Autodesk Fusion 360 part; units mm, degrees
sketch "Sketch1" plane through (0, 0, 0) normal (0, 1, 0) x (1, 0, 0)
  line L0 (0, 0) -> (79, 0)
  line L1 (79, 0) -> (79, -80)
  line L2 (79, -80) -> (0, -80)
  line L3 (0, -80) -> (0, 0)
  dimension "d1" = 79
  dimension "d2" = 80
extrude "Extrude1" add sketch "Sketch1" along normal blind 5
sketch "Sketch2" plane through (0, 5, 0) normal (0, 1, 0) x (-1, 0, 0)
  line L0 (0, 80) -> (-79, 80)
  line L1 (-79, 80) -> (-79, 0)
  line L2 (-79, 0) -> (0, 0)
  line L3 (0, 0) -> (0, 80)
  point P0 (-14, 77.5)
  dimension "d5" = 14
  dimension "d6" = 2.5
hole "Hole1" at (14, 5, 77.5) direction (0, -1, 0) diameter 2 end through all counterbore diameter 4.4 counterbore depth 2.2
pattern_linear "R-Pattern1" count 1 spacing 0 along (0, 0, -1) count 4 spacing 17 along (1, 0, 0) of "Hole1"
Model file for the job. Use its own axes, mm. A direction names the side the tool comes from. Round coordinates to 2 decimals unless told otherwise and drop trailing zeros. Write each loop counter-clockwise with the first axis right and the second up, starting at its lowest first coordinate (ties: lowest second). Pieces come first, ordered by that corner, then holes. Notation, with made-up numbers: (39, 38.5) - (43, 38.5) arc R16 cw to (43, 61.5) - close; hole circle Ø5 at (61, 16). An arc over 180 degrees is marked (long way). One line per item, written item: value.
(1) Two-plate mould, pull along Z, no slides. Class faces 1 (the flat face through (79, 2, 39)), 2 (the cylindrical face through (47.324, 1.38, 76.763)), 3 (the flat face through (40, 2, 80)): pulls with the +Z half, pulls with the -Z half, needs draft (parallel to the pull), parting line crosses it, or undercut.
Values follow:
face 1: needs draft
face 2: undercut
face 3: pulls with the +Z half
(2) Cut at B-B, the plane z = 77.5. Give the number of separate pieces and of enclosed holes in the cut face, plus the area to 3 significant figures.
Values follow:
separate pieces: 5
enclosed holes: 0
area: 334 mm²
(3) Drop flat-ended pins along their axis: P1, Ø3, axis at x = 60, y = 3.5, coming from the -Z side; P2, Ø1.6, axis at x = 48, z = 77.5, coming from the -Y side; P3, Ø1.3, axis at x = 30.5, z = 78.5, coming from the +Y side. Give the stop position or say it passes through.
Values follow:
P1: stops at z = 0
P2: passes through
P3: stops at y = 2.8
(4) Cut at A-A, the plane x = 48. Give the cut face in (y, z), plus the area to 3 significant figures.
Values follow:
outline: (0, 0) - (5, 0) - (5, 75.3) - (2.8, 75.3) - (2.8, 76.5) - (0, 76.5) - close; (0, 78.5) - (2.8, 78.5) - (2.8, 79.7) - (5, 79.7) - (5, 80) - (0, 80) - close
area: 385 mm²
(5) Wall check: probe 1 along X at (y, z) = (1.3, 77.5); probe 2 along X at (y, z) = (3.9, 77.5); probe 3 along Z at (x, y) = (14, 3.9). Give the ranges that are in metal, low to high.
Values follow:
probe 1: x = 0 to 13, 15 to 30, 32 to 47, 49 to 64, 66 to 79
probe 2: x = 0 to 11.8, 16.2 to 28.8, 33.2 to 45.8, 50.2 to 62.8, 67.2 to 79
probe 3: z = 0 to 75.3, 79.7 to 80
(6) 3-axis set-ups, long thin cutter, end or side, ignore diameter. For faces 4 (the flat face through (39, 0, 39)), 5 (the cylindrical face through (13.34, 3.88, 79.6)): which of +Z, -Z, +X, -X, +Y, -Y reach the whole face in a straight line?
Values follow:
face 4: +Z, -Z, +X, -X, -Y
face 5: +Y
